from build123d import *

# Parameters (mm, degrees)
F1_DEPTH = 3.81
F4_DEPTH = 71.628
F6_DEPTH = 1.27
F7_R     = 1.778
F8_DEPTH = 5.842
F9_R     = 5.08


with BuildPart() as f1:
    # F0 (on Front) → F1 (new body)
    with BuildSketch(Plane.XZ):
        Polygon((-38.4448663006, 16.8945933835), (-38.4448663006, 14.7355933835), (33.1831336994, 14.7355933835), (33.1831336994, 16.8945933835), (28.6111336994, 16.8945933835), (27.0871336994, 16.8945933835), (22.5151336994, 16.8945933835), (20.9911336994, 16.8945933835), (16.4191336994, 16.8945933835), (14.8951336994, 16.8945933835), (10.3231336994, 16.8945933835), (8.7991336994, 16.8945933835), (4.2271336994, 16.8945933835), (2.7031336994, 16.8945933835), (-1.8688663006, 16.8945933835), (-3.3928663006, 16.8945933835), (-7.9648663006, 16.8945933835), (-9.4888663006, 16.8945933835), (-14.0608663006, 16.8945933835), (-15.5848663006, 16.8945933835), (-20.1568663006, 16.8945933835), (-21.6808663006, 16.8945933835), (-26.2528663006, 16.8945933835), (-27.7768663006, 16.8945933835), (-32.3488663006, 16.8945933835), (-33.8728663006, 16.8945933835), align=None)
        Polygon((-37.1748663006, 21.2125933835), (-38.4448663006, 16.8945933835), (-33.8728663006, 16.8945933835), (-35.1428663006, 21.2125933835), align=None)
        Polygon((28.6111336994, 16.8945933835), (33.1831336994, 16.8945933835), (31.9131336994, 21.2125933835), (29.8811336994, 21.2125933835), align=None)
        Polygon((-31.0788663006, 21.2125933835), (-32.3488663006, 16.8945933835), (-27.7768663006, 16.8945933835), (-29.0468663006, 21.2125933835), align=None)
        Polygon((22.5151336994, 16.8945933835), (27.0871336994, 16.8945933835), (25.8171336994, 21.2125933835), (23.7851336994, 21.2125933835), align=None)
        Polygon((-24.9828663006, 21.2125933835), (-26.2528663006, 16.8945933835), (-21.6808663006, 16.8945933835), (-22.9508663006, 21.2125933835), align=None)
        Polygon((16.4191336994, 16.8945933835), (20.9911336994, 16.8945933835), (19.7211336994, 21.2125933835), (17.6891336994, 21.2125933835), align=None)
        Polygon((-18.8868663006, 21.2125933835), (-20.1568663006, 16.8945933835), (-15.5848663006, 16.8945933835), (-16.8548663006, 21.2125933835), align=None)
        Polygon((10.3231336994, 16.8945933835), (14.8951336994, 16.8945933835), (13.6251336994, 21.2125933835), (11.5931336994, 21.2125933835), align=None)
        Polygon((-12.7908663006, 21.2125933835), (-14.0608663006, 16.8945933835), (-9.4888663006, 16.8945933835), (-10.7588663006, 21.2125933835), align=None)
        Polygon((4.2271336994, 16.8945933835), (8.7991336994, 16.8945933835), (7.5291336994, 21.2125933835), (5.4971336994, 21.2125933835), align=None)
        Polygon((-6.6948663006, 21.2125933835), (-7.9648663006, 16.8945933835), (-3.3928663006, 16.8945933835), (-4.6628663006, 21.2125933835), align=None)
        Polygon((-1.8688663006, 16.8945933835), (2.7031336994, 16.8945933835), (1.4331336994, 21.2125933835), (-0.5988663006, 21.2125933835), align=None)
    extrude(amount=F1_DEPTH)

    # F3 (on plane+point) → F4 (join, through all)
    with BuildSketch(Plane.YZ.offset(33.1831336994)):
        Polygon((-15.494, 14.7355933835), (-3.81, 14.7355933835), (-3.81, 16.8945933835), (-7.874, 16.8945933835), (-7.874, 19.0535933835), (-11.684, 19.0535933835), (-11.684, 16.8945933835), (-15.494, 16.8945933835), align=None)
    extrude(amount=-F4_DEPTH)

    # F5 (on face) → F6 (join)
    with BuildSketch(Plane(origin=(0, 0, 0), x_dir=(-1, 0, 0), z_dir=(0, 1, 0))):
        Polygon((33.8728663006, 16.8945933835), (35.1428663006, 21.2125933835), (31.0788663006, 21.2125933835), (32.3488663006, 16.8945933835), align=None)
        Polygon((27.7768663006, 16.8945933835), (29.0468663006, 21.2125933835), (24.9828663006, 21.2125933835), (26.2528663006, 16.8945933835), align=None)
        Polygon((21.6808663006, 16.8945933835), (22.9508663006, 21.2125933835), (18.8868663006, 21.2125933835), (20.1568663006, 16.8945933835), align=None)
        Polygon((15.5848663006, 16.8945933835), (16.8548663006, 21.2125933835), (12.7908663006, 21.2125933835), (14.0608663006, 16.8945933835), align=None)
        Polygon((9.4888663006, 16.8945933835), (10.7588663006, 21.2125933835), (6.6948663006, 21.2125933835), (7.9648663006, 16.8945933835), align=None)
        Polygon((3.3928663006, 16.8945933835), (4.6628663006, 21.2125933835), (0.5988663006, 21.2125933835), (1.8688663006, 16.8945933835), align=None)
        Polygon((-1.4331336994, 21.2125933835), (-5.4971336994, 21.2125933835), (-4.2271336994, 16.8945933835), (-2.7031336994, 16.8945933835), align=None)
        Polygon((-7.5291336994, 21.2125933835), (-11.5931336994, 21.2125933835), (-10.3231336994, 16.8945933835), (-8.7991336994, 16.8945933835), align=None)
        Polygon((-13.6251336994, 21.2125933835), (-17.6891336994, 21.2125933835), (-16.4191336994, 16.8945933835), (-14.8951336994, 16.8945933835), align=None)
        Polygon((-19.7211336994, 21.2125933835), (-23.7851336994, 21.2125933835), (-22.5151336994, 16.8945933835), (-20.9911336994, 16.8945933835), align=None)
        Polygon((-25.8171336994, 21.2125933835), (-29.8811336994, 21.2125933835), (-28.6111336994, 16.8945933835), (-27.0871336994, 16.8945933835), align=None)
        Polygon((-33.1831336994, 14.7355933835), (38.4448663006, 14.7355933835), (38.4448663006, 16.8945933835), (37.1748663006, 21.2125933835), (35.1428663006, 21.2125933835), (33.8728663006, 16.8945933835), (32.3488663006, 16.8945933835), (31.0788663006, 21.2125933835), (29.0468663006, 21.2125933835), (27.7768663006, 16.8945933835), (26.2528663006, 16.8945933835), (24.9828663006, 21.2125933835), (22.9508663006, 21.2125933835), (21.6808663006, 16.8945933835), (20.1568663006, 16.8945933835), (18.8868663006, 21.2125933835), (16.8548663006, 21.2125933835), (15.5848663006, 16.8945933835), (14.0608663006, 16.8945933835), (12.7908663006, 21.2125933835), (10.7588663006, 21.2125933835), (9.4888663006, 16.8945933835), (7.9648663006, 16.8945933835), (6.6948663006, 21.2125933835), (4.6628663006, 21.2125933835), (3.3928663006, 16.8945933835), (1.8688663006, 16.8945933835), (0.5988663006, 21.2125933835), (-1.4331336994, 21.2125933835), (-2.7031336994, 16.8945933835), (-4.2271336994, 16.8945933835), (-5.4971336994, 21.2125933835), (-7.5291336994, 21.2125933835), (-8.7991336994, 16.8945933835), (-10.3231336994, 16.8945933835), (-11.5931336994, 21.2125933835), (-13.6251336994, 21.2125933835), (-14.8951336994, 16.8945933835), (-16.4191336994, 16.8945933835), (-17.6891336994, 21.2125933835), (-19.7211336994, 21.2125933835), (-20.9911336994, 16.8945933835), (-22.5151336994, 16.8945933835), (-23.7851336994, 21.2125933835), (-25.8171336994, 21.2125933835), (-27.0871336994, 16.8945933835), (-28.6111336994, 16.8945933835), (-29.8811336994, 21.2125933835), (-31.9131336994, 21.2125933835), (-33.1831336994, 16.8945933835), align=None)
        Polygon((37.1748663006, 21.2125933835), (38.4448663006, 16.8945933835), (38.4448663006, 21.2125933835), align=None)
    extrude(amount=F6_DEPTH)

    # F7 (on face) → F8 (join)
    with BuildSketch(Plane(origin=(0, 1.27, 0), x_dir=(-1, 0, 0), z_dir=(0, 1, 0))):
        Polygon((38.4448663006, 14.7355933835), (38.4448663006, 21.2125933835), (38.4448663006, 40.5165933835), (26.5068663006, 40.5165933835), (26.5068663006, 14.7355933835), align=None)
        with Locations((29.6818663006, 23.4985933835)):
            Circle(F7_R, mode=Mode.SUBTRACT)
        with Locations((29.6818663006, 36.1985933835)):
            Circle(F7_R, mode=Mode.SUBTRACT)
    extrude(amount=F8_DEPTH)

    # F9
    f9_edges = [f1.edges().sort_by_distance(p)[0] for p in [
        (-38.444866, 4.191, 40.516593),
    ]]
    fillet(f9_edges, radius=F9_R)


solid = f1.part
The listing builds one solid part. Answer for the finished solid, in the listing's coordinates (mm). A direction names the side the tool comes from. Give positions to 0.01 mm unless a question says otherwise; leave off trailing zeros. Order: outer loops, then holes, each group sorted by start corner. A loop starts at its lowest first (then second) coordinate and runs counter-clockwise, first axis right, second up. Notation, with made-up numbers: (5.25, 79.25) - (43.25, 79.25) arc R31 cw to (43.25, 106.25) - close; hole circle Ø6 at (55.5, -25). An arc over 180 degrees is marked (long way). Use one line per item in the form item = value.
1) For faces 1 (the flat face through (-38, 0, 20)), 2 (the cylindrical face through (-30.5, 4.15, 21.92)), 3 (the flat face through (-32, 1.27, 31)), 4 (the flat face through (-26.507, 4, 28)), 5 (the flat face through (-22.3, -1.9, 19)), determine the directions among +Z, -Z, +X, -X, +Y, -Y from which every point of the face is accessible in a straight line to the end or side of a thin tool.
Verdict:
face_1 = +Z, -X
face_2 = +Y, -Y
face_3 = +Z, +X, -X, -Y
face_4 = +Z, -Z, +X, +Y
face_5 = +Z
2) Find section D-D on y = -13. Determine the outline of the cut face in (x, z), and give its area (3 significant figures).
Verdict:
outline = (-38.44, 14.74) - (33.18, 14.74) - (33.18, 16.89) - (-38.44, 16.89) - close
area = 155 mm^2
3) The mould has two halves that part along X. Classify faces 6 (the flat face through (-7.321, -1.878, 19.084)), 7 (the flat face through (-33, 0, 20)), 8 (the cylindrical face through (-36.996, 4.232, 38.989)), 9 (the flat face through (-12, -3.81, 19)): released by +X, released by -X, zero draft, split by the parting line, or undercut.
Verdict:
face_6 = undercut
face_7 = undercut
face_8 = released by -X
face_9 = zero draft
4) Find section A-A on x = -18. Determine the outline of the cut face in (y, z).
Verdict:
outline = (-15.49, 14.74) - (1.27, 14.74) - (1.27, 21.21) - (-3.81, 21.21) - (-3.81, 16.89) - (-7.87, 16.89) - (-7.87, 19.05) - (-11.68, 19.05) - (-11.68, 16.89) - (-15.49, 16.89) - close
5) Find section C-C on y = 2.5. Determine the outline of the cut face in (x, z).
Verdict:
outline = (-38.44, 14.74) - (-26.51, 14.74) - (-26.51, 40.52) - (-33.36, 40.52) arc R5.08 ccw to (-38.44, 35.44) - close; hole circle Ø3.56 at (-29.68, 23.5); hole circle Ø3.56 at (-29.68, 36.2)
6) Each of these flat-tipped pins is pushed along its axis until it touches: pin 1 (1.5 mm diameter, centred on y = -2, z = 18.5, fed in from -X); pin 2 (1.3 mm diameter, centred on x = 25.5, z = 19.5, fed in from -Y); pin 3 (1.4 mm diameter, centred on x = -37.5, z = 20, fed in from -Y). Where does it stop, or does it pass through?
Verdict:
pin_1 = -38.19
pin_2 = -11.68
pin_3 = -3.81
7) Find section B-B on z = 24.5. Determine the outline of the cut face in (x, y), and give its area (3 significant figures).
Verdict:
outline = (-38.44, 1.27) - (-31.15, 1.27) - (-31.15, 7.11) - (-38.44, 7.11) - close; (-28.21, 1.27) - (-26.51, 1.27) - (-26.51, 7.11) - (-28.21, 7.11) - close
area = 52.6 mm^2
8) Consider probe 1 along Y at (x, z) = (15, 19); probe 2 along Y at (x, z) = (-13, 18.5); probe 3 along X at (y, z) = (4.5, 27.5). Determine where each line is inside the solid, lowest interval first. Write a range as [from, to].
Verdict:
probe_1 = [-11.68, -7.87], [0, 1.27]
probe_2 = [-11.68, -7.87], [-3.81, 1.27]
probe_3 = [-38.44, -26.51]
